Part model, mm, in its own coordinate system. Face numbers are marked on the shaded views. A direction names the side the tool comes from. Coordinates: 2 decimals unless noted, no trailing zeros. Answer as a JSON object with one key per item and string values. Group by question number.
1. 3-axis set-ups, long thin cutter, end or side, ignore diameter. For the marked faces 1 and 2: which of +Z, -Z, +X, -X, +Y, -Y reach the whole face in a straight line?
2. Drop flat-ended pins along their axis: pin 1 Ø1.5 at (x, y) = (-3, 27.5) entering from -Z; pin 2 Ø5 at (x, z) = (-5.5, -3.5) entering from -Y; pin 3 Ø3.5 at (x, z) = (-2, 0.5) entering from -Y. Give the stop position or say it passes through.
3. Drill centre lines: L1, parallel to Y at x = -5.5, z = -2; L2, parallel to X at y = 26.5, z = -2; L3, parallel to Y at x = 6.75, z = -2.75. Where is each one in solid material? Low to high.
4. Saw through at A-A on z = 1.25. Count the separate pieces of the cut face and the enclosed holes in it, then the cut area to 3 significant figures.
5. Mould opens along Y. For the marked faces 3, 4 and 5 say: released by +Y, released by -Y, zero draft, split by the parting line, or undercut.
from build123d import *

# Parameters (mm, degrees)
FILLET1_R               = 1
SKETCH2_W               = 2
SKETCH2_H               = 3
CUT_REVOLVE1_ANGLE      = 180
CUT_EXTRUDE1_REACH      = 45.319
CUT_EXTRUDE1_END_RADIUS = 7.5
SKETCH2_3_W             = 2
SKETCH2_3_H             = 3
CUT_EXTRUDE2_REACH      = 32.879
FILLET2_R               = 0.5
FILLET3_R               = 5


with BuildPart() as part:
    # Sketch1 → Revolve1 (revolve)
    with BuildSketch(Plane.XY, mode=Mode.PRIVATE) as revolve1_sk:
        with BuildLine():
            Line((2.4, 42), (2.4, 0))
            Line((2.4, 0), (4.4, 0))
            Line((4.4, 0), (4.4, 1.75))
            ThreePointArc((4.4, 1.75), (4.55, 2.75), (4.4, 3.75))
            Line((4.4, 3.75), (4.4, 5.5))
            ThreePointArc((4.4, 5.5), (4.55, 6.5), (4.4, 7.5))
            Line((4.4, 7.5), (4.4, 9.25))
            ThreePointArc((4.4, 9.25), (4.55, 10.25), (4.4, 11.25))
            Line((4.4, 11.25), (4.4, 13))
            Line((4.4, 13), (7.5, 13))
            Line((7.5, 13), (7.5, 18))
            Line((7.5, 18), (4.7, 18))
            Line((4.7, 18), (4.7, 22))
            Line((4.7, 22), (5.717261497, 22))
            Line((5.717261497, 22), (4.7, 27))
            Line((4.7, 27), (5.717261497, 27))
            Line((5.717261497, 27), (4.7, 32))
            Line((4.7, 32), (5.717261497, 32))
            Line((5.717261497, 32), (4.7, 37))
            Line((4.7, 37), (5.717261497, 37))
            Line((5.717261497, 37), (4.7, 42))
            Line((4.7, 42), (2.4, 42))
        make_face()
    revolve(revolve1_sk.sketch.rotate(Axis((0, 7.836928881, 0), (0, 1, 0)), 90), axis=Axis((0, 7.836928881, 0), (0, 1, 0)))

    # Fillet1
    fillet1_edges = [part.edges().sort_by_distance(p)[0] for p in [
        (0, 42, 4.7),
    ]]
    fillet(fillet1_edges, radius=FILLET1_R)

    # Sketch2 → Cut-Revolve1 (revolve, cut)
    with BuildSketch(Plane.XY):
        with Locations((5.7, 15.5)):
            Rectangle(SKETCH2_W, SKETCH2_H)
    revolve(axis=Axis((0, 0, 0), (0, 1, 0)), revolution_arc=CUT_REVOLVE1_ANGLE, mode=Mode.SUBTRACT)

    # Cut-Extrude1: up to this cylinder (the profile starts inside it)
    cut_extrude1_end = Plane(origin=(0, 15.5, 0), z_dir=(0, -1, 0)) * Cylinder(CUT_EXTRUDE1_END_RADIUS, 106.638, mode=Mode.PRIVATE)
    # Sketch2<3> → Cut-Extrude1 (cut, up to the surface)
    with BuildSketch(Plane.XY, mode=Mode.PRIVATE) as cut_extrude1_sk1:
        with Locations((-5.7, 15.5)):
            Rectangle(SKETCH2_3_W, SKETCH2_3_H)
    cut_extrude1_tool1 = extrude(cut_extrude1_sk1.sketch, amount=CUT_EXTRUDE1_REACH, mode=Mode.PRIVATE) & cut_extrude1_end
    add(cut_extrude1_tool1.solids().sort_by_distance((-5.7, 15.5, 0))[0], mode=Mode.SUBTRACT)
    # Sketch2<3> → Cut-Extrude1 (cut, up to the surface)
    with BuildSketch(Plane.XY, mode=Mode.PRIVATE) as cut_extrude1_sk2:
        with Locations((5.7, 15.5)):
            Rectangle(SKETCH2_3_W, SKETCH2_3_H)
    cut_extrude1_tool2 = extrude(cut_extrude1_sk2.sketch, amount=CUT_EXTRUDE1_REACH, mode=Mode.PRIVATE) & cut_extrude1_end
    add(cut_extrude1_tool2.solids().sort_by_distance((5.7, 15.5, 0))[0], mode=Mode.SUBTRACT)

    # Sketch3 → Cut-Extrude2 (cut, up to next)
    with BuildSketch(Plane.XZ.offset(-13), mode=Mode.PRIVATE) as cut_extrude2_sk1:
        with BuildLine():
            Line((3.066054247, 6.844655678), (-3.066054247, 6.844655678))
            ThreePointArc((-3.066054247, 6.844655678), (0, 7.5), (3.066054247, 6.844655678))
        make_face()
    cut_extrude2_tool1 = extrude(cut_extrude2_sk1.sketch, amount=-CUT_EXTRUDE2_REACH, mode=Mode.PRIVATE) & part.part
    add(cut_extrude2_tool1.solids().sort_by_distance((0, 13, 7.107801))[0], mode=Mode.SUBTRACT)

    # Fillet2
    fillet2_edges = [part.edges().sort_by_distance(p)[0] for p in [
        (0, 0, 4.4),
    ]]
    fillet(fillet2_edges, radius=FILLET2_R)

    # Fillet3
    # the kernel refuses this fillet: 5 mm, written as the material it takes off along each edge
    with BuildSketch(Plane(origin=(0, 0, 0), x_dir=(0, 0, -1), z_dir=(1, 0, 0))) as fillet3_piece_1:
        with BuildLine():
            CenterArc((7.4, 3.570714214), FILLET3_R, 180, 45.572995999)
            Line((2.4, 3.570714214), (2.4, 0))
            Line((2.4, 0), (3.9, 0))
        make_face()
    revolve(axis=Axis((0, 0, 0), (0, 1, 0)), mode=Mode.SUBTRACT)
    with BuildSketch(Plane(origin=(0, 42, 0), x_dir=(0, 0, -1), z_dir=(1, 0, 0))) as fillet3_piece_2:
        with BuildLine():
            CenterArc((7.4, -3.553937245), FILLET3_R, 134.700979484, 45.299020516)
            Line((3.88296573, 0), (2.4, 0))
            Line((2.4, 0), (2.4, -3.553937245))
        make_face()
    revolve(axis=Axis((0, 42, 0), (0, 1, 0)), mode=Mode.SUBTRACT)


solid = part.part
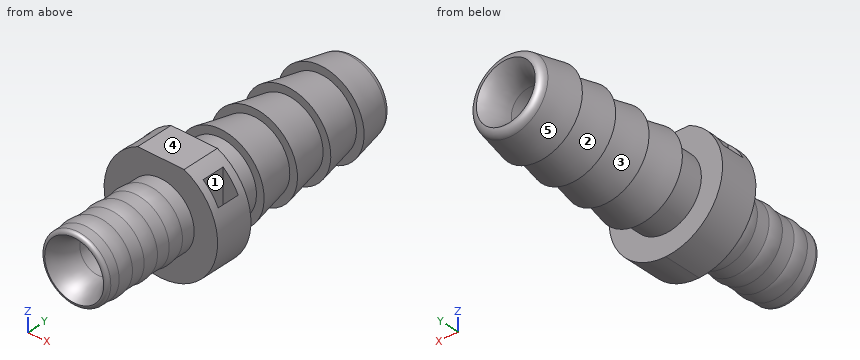
Outcome:
{
 "1": {"face 1": "+Z", "face 2": "none"},
 "2": {"pin 1": "stops at z = -5.18", "pin 2": "stops at y = 0.01", "pin 3": "stops at y = 0.09"},
 "3": {"L1": "y = 13 to 14, 17 to 18", "L2": "x = -4.37 to -1.33, 1.33 to 4.37", "L3": "y = 13 to 18"},
 "4": {"separate pieces": "2", "enclosed holes": "2", "area": "231 mm²"},
 "5": {"face 3": "undercut", "face 4": "zero draft", "face 5": "released by +Y"}
}
